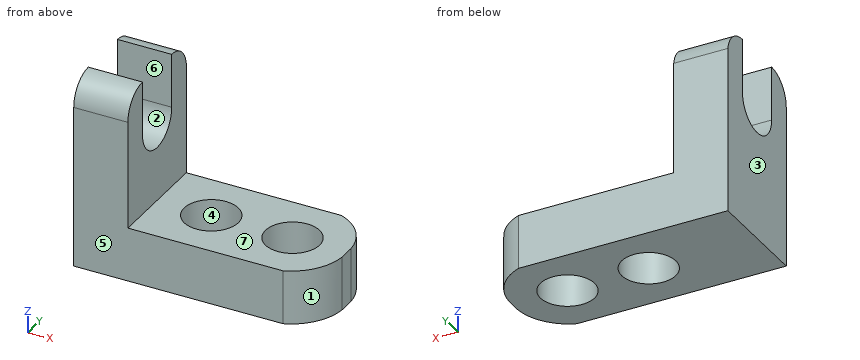
```python
from build123d import *

# Parameters (mm, degrees)
F1_DEPTH = 25.4
F3_DEPTH = 25.4
F5_DEPTH = 25.4
F6_R     = 6.35
F7_DEPTH = 25.4
F9_DEPTH = 25.4


with BuildPart() as f1:
    # F0 (on Front) → F1 (new body)
    with BuildSketch(Plane.XZ):
        Polygon((0, 44.45), (0, 0), (57.15, 0), (57.15, 12.7), (12.7, 12.7), (12.7, 44.45), align=None)
    extrude(amount=F1_DEPTH)

    # F2 (on face) → F3 (cut)
    with BuildSketch(Plane.YZ.offset(12.7)):
        with BuildLine():
            ThreePointArc((-19.05, 31.75), (-12.7, 25.4), (-6.35, 31.75))
            ThreePointArc((-6.35, 31.75), (-12.7, 38.1), (-19.05, 31.75))
        make_face()
        with BuildLine():
            ThreePointArc((-19.05, 31.75), (-12.7, 38.1), (-6.35, 31.75))
            Line((-6.35, 31.75), (-6.35, 44.45))
            Line((-6.35, 44.45), (-19.05, 44.45))
            Line((-19.05, 44.45), (-19.05, 31.75))
        make_face()
    extrude(amount=-F3_DEPTH, mode=Mode.SUBTRACT)

    # F4 (on face) → F5 (cut)
    with BuildSketch(Plane.YZ.offset(12.7)):
        with BuildLine():
            Line((-25.4, 44.45), (-25.4, 38.1))
            ThreePointArc((-25.4, 38.1), (-23.540128, 42.590128), (-19.05, 44.45))
            Line((-19.05, 44.45), (-25.4, 44.45))
        make_face()
        with BuildLine():
            Line((0, 44.45), (-6.35, 44.45))
            ThreePointArc((-6.35, 44.45), (-2.156385, 42.890804), (0, 38.970664))
            Line((0, 38.970664), (0, 44.45))
        make_face()
    extrude(amount=-F5_DEPTH, mode=Mode.SUBTRACT)

    # F6 (on face) → F7 (cut)
    with BuildSketch(Plane.XY.offset(12.7)):
        with Locations((44.45, -12.7)):
            Circle(F6_R)
        with Locations((25.4, -12.7)):
            Circle(F6_R)
    extrude(amount=-F7_DEPTH, mode=Mode.SUBTRACT)

    # F8 (on face) → F9 (cut)
    with BuildSketch(Plane.XY.offset(12.7)):
        with BuildLine():
            Line((57.15, -25.4), (57.15, -14.733049))
            ThreePointArc((57.15, -14.733049), (54.656516, -21.24776), (49.051356, -25.4))
            Line((49.051356, -25.4), (57.15, -25.4))
        make_face()
        with BuildLine():
            ThreePointArc((57.15, -14.733049), (57.191553, -13.716524), (57.15, -12.7))
            Line((57.15, -12.7), (57.15, -14.733049))
        make_face()
        with BuildLine():
            ThreePointArc((57.15, -12.7), (57.186039, -11.749483), (57.15, -10.798966))
            Line((57.15, -10.798966), (57.15, -12.7))
        make_face()
        with BuildLine():
            Line((57.15, 0), (49.051356, 0))
            ThreePointArc((49.051356, 0), (54.675771, -4.218247), (57.15, -10.798966))
            Line((57.15, -10.798966), (57.15, 0))
        make_face()
    extrude(amount=-F9_DEPTH, mode=Mode.SUBTRACT)


solid = f1.part
```
Geometry: final body of the model. Coordinates: model frame, mm. Face numbers are marked on the shaded views. A direction names the side the tool comes from. Coordinates: 2 decimals unless noted, no trailing zeros. Loops run counter-clockwise (first coordinate to the right, second up) from the corner with the lowest first, then second, coordinate; pieces in that order, holes last. Notation, with made-up numbers: M 81.25,33 L 131.25,33 A11 cw 131.25,42 Z; hole C -12.5,24 d10. An arc over 180 degrees is marked long. Put each result on its own line as item: value.
(1) Material intervals for probe 1 along Y at (x, z) = (44.45, 5); probe 2 along Z at (x, y) = (16.5, -8), sorted ascending.
Answer sheet:
probe 1: y = -25.4 to -19.05, -6.35 to 0
probe 2: z = 0 to 12.7
(2) Cut plane B-B on y = -18. Return the cut outline in (x, z), then the cut area to 3 significant figures.
Answer sheet:
outline: M 0,0 L 21.9,0 L 21.9,12.7 L 12.7,12.7 L 12.7,28.25 L 0,28.25 Z; M 28.9,0 L 40.95,0 L 40.95,12.7 L 28.9,12.7 Z; M 47.95,0 L 56.43,0 L 56.43,12.7 L 47.95,12.7 Z
area: 737 mm^2
(3) First-contact query: pin 1 (12 mm diameter, centred on x = 34.5, z = 24.5, fed in from +Y); pin 2 (5 mm diameter, centred on y = -6, z = 32, fed in from +X). Flat tips, straight axial feed; report the tip coordinate or a pass-through.
Answer sheet:
pin 1: passes through
pin 2: stops at x = 12.7
(4) Access query for the marked faces 5, 6 and 7. Directions: +Z, -Z, +X, -X, +Y, -Y. A direction counts if a zero-diameter tool reaches every point of the face in a straight line with its end or side. Return the directions, or none.
Answer sheet:
face 5: +Z, -Z, +X, -X, -Y
face 6: +Z, +X, -X
face 7: +Z, +X, +Y, -Y
(5) Cut plane D-D on x = 5.5. Return the cut outline in (y, z), then the cut area to 3 significant figures.
Answer sheet:
outline: M -25.4,0 L 0,0 L 0,38.97 A6.42 ccw -6.35,44.45 L -6.35,31.75 A6.35 cw -19.05,31.75 L -19.05,44.45 A6.35 ccw -25.4,38.1 Z
area: 887 mm^2
(6) Cut plane C-C on z = 28. Return the cut outline in (x, y), then the cut area to 3 significant figures.
Answer sheet:
outline: M 0,-25.4 L 12.7,-25.4 L 12.7,-17.82 L 0,-17.82 Z; M 0,-7.58 L 12.7,-7.58 L 12.7,0 L 0,0 Z
area: 192 mm^2
(7) Cut plane A-A on x = 44.45. Return the cut outline in (y, z), then the cut area to 3 significant figures.
Answer sheet:
outline: M -25.4,0 L -19.05,0 L -19.05,12.7 L -25.4,12.7 Z; M -6.35,0 L 0,0 L 0,12.7 L -6.35,12.7 Z
area: 161 mm^2
(8) Draft query along Y for the marked faces 1, 2, 3 and 4. Return one class per face: pulls with the +Y half, pulls with the -Y half, needs draft (parallel to the pull), parting line crosses it, or undercut.
Answer sheet:
face 1: pulls with the -Y half
face 2: undercut
face 3: needs draft
face 4: undercut
